Here's how the part is built. I have some questions about the finished solid (model axes, mm). Face numbers are marked on the shaded views. A direction names the side the tool comes from. Round coordinates to 2 decimals unless told otherwise and drop trailing zeros. Write each loop counter-clockwise with the first axis right and the second up, starting at its lowest first coordinate (ties: lowest second). Pieces come first, ordered by that corner, then holes. Notation, with made-up numbers: (6.5, 80.5) -> (60.5, 80.5) arc R16 cw to (60.5, 105.5) -> close; hole circle Ø5 at (76, 57). An arc over 180 degrees is marked (long way). Put each result on its own line as item: value. Start each with the question number.
1) I want a section at B-B, the plane z = -15.5. List the corners of the cut face in (x, y) for me.
2) I want a section at A-A, the plane x = 15.5. List the corners of the cut face in (y, z) for me, then the cut area to 3 significant figures.
3) Which directions (+Z, -Z, +X, -X, +Y, -Y) give clear straight access to the entire face, cutting with the end or side of a thin tool? Please do the marked faces 1, 2 and 3.
4) I want a section at C-C, the plane y = 3.4. List the corners of the cut face in (x, z) for me.
5) If I drill on line 1 along Z through (x, y) = (7.5, 3.2); line 2 along Z through (x, y) = (7.5, 1.75); line 3 along X through (y, z) = (2.9, -55), over which ranges is the centre line in solid material (lowest first)? Write a range as [from, to].
6) Will these pins go through, and if not, where does the flat tip stop? P1, Ø6, axis at x = 22.5, z = -40, coming from the +Y side; P2, Ø3, axis at y = 1.5, z = -19, coming from the -X side; P3, Ø1.2, axis at x = 2.5, y = 3.5, coming from the +Z side.
7) I want a section at D-D, the plane z = -55. List the corners of the cut face in (x, y) for me.
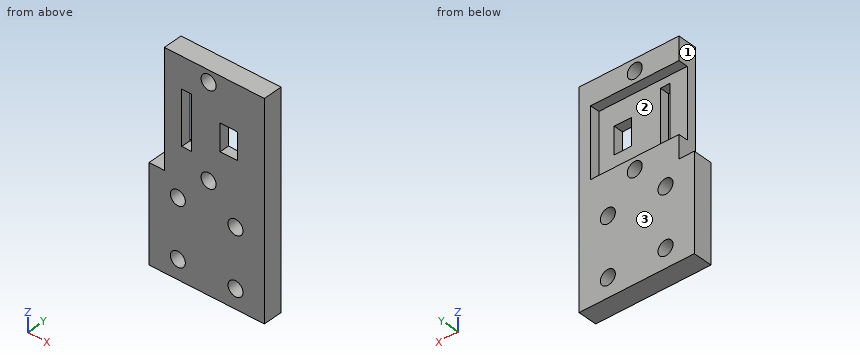
from build123d import *

# Parameters (mm, degrees)
ESQUISSE1_W             = 30
ESQUISSE1_H             = 60
BOSS_EXTRU_1_DEPTH      = 5
D_GAGEMENT_M3_51_D      = 3.9
ESQUISSE19_W            = 26
ESQUISSE19_H            = 5
ENL_V_MAT_EXTRU_5_DEPTH = 6
D_GAGEMENT_M3_53_D      = 3.9
D_GAGEMENT_M3_53_DEPTH  = 5
D_GAGEMENT_M3_53_TIP    = 1.171678207
ESQUISSE22_W            = 23
ESQUISSE22_H            = 18
ENL_V_MAT_EXTRU_6_DEPTH = 2.5
ESQUISSE23_W            = 2.5
ESQUISSE23_H            = 14
ESQUISSE23_W_2          = 4.5
ESQUISSE23_H_2          = 7
ENL_V_MAT_EXTRU_7_DEPTH = 3.5


with BuildPart() as part:
    # Esquisse1 → Boss.-Extru.1 (new body)
    with BuildSketch(Plane(origin=(0, 0, 0), x_dir=(1, 0, 0), z_dir=(0, 1, 0))):
        with Locations((15, 30)):
            Rectangle(ESQUISSE1_W, ESQUISSE1_H)
    extrude(amount=BOSS_EXTRU_1_DEPTH)

    # Dégagement M3.51 (through all)
    with Locations(Plane(origin=(0, 5, 0), x_dir=(1, 0, 0), z_dir=(0, 1, 0))):
        with Locations((7.5, 40), (22.5, 40), (22.5, 55), (7.5, 55)):
            Hole(D_GAGEMENT_M3_51_D / 2)

    # Esquisse19 → Enlèv. mat.-Extru.5 (cut, through all)
    with BuildSketch(Plane(origin=(0, 5, 0), x_dir=(1, 0, 0), z_dir=(0, 1, 0))):
        Polygon((4, 5), (4, 35), (0, 35), (0, 0), (4, 0), align=None)
        with Locations((17, 2.5)):
            Rectangle(ESQUISSE19_W, ESQUISSE19_H)
    extrude(amount=-ENL_V_MAT_EXTRU_5_DEPTH, mode=Mode.SUBTRACT)

    # Dégagement M3.53
    with Locations(Plane(origin=(0, 5, 0), x_dir=(1, 0, 0), z_dir=(0, 1, 0))):
        with Locations((15.5, 32), (15.5, 8)):
            Hole(D_GAGEMENT_M3_53_D / 2, depth=D_GAGEMENT_M3_53_DEPTH)
            with Locations((0, 0, -(D_GAGEMENT_M3_53_DEPTH + D_GAGEMENT_M3_53_TIP / 2))):  # 118° drill point
                Cone(0, D_GAGEMENT_M3_53_D / 2, D_GAGEMENT_M3_53_TIP, mode=Mode.SUBTRACT)

    # Esquisse22 → Enlèv. mat.-Extru.6 (cut)
    with BuildSketch(Plane(origin=(0, 5, 0), x_dir=(1, 0, 0), z_dir=(0, 1, 0))):
        with Locations((15.5, 20)):
            Rectangle(ESQUISSE22_W, ESQUISSE22_H)
    extrude(amount=-ENL_V_MAT_EXTRU_6_DEPTH, mode=Mode.SUBTRACT)

    # Esquisse23 → Enlèv. mat.-Extru.7 (cut, through all)
    with BuildSketch(Plane(origin=(0, 2.5, 0), x_dir=(1, 0, 0), z_dir=(0, 1, 0))):
        with Locations((9.75, 20)):
            Rectangle(ESQUISSE23_W, ESQUISSE23_H)
        with Locations((20.75, 20)):
            Rectangle(ESQUISSE23_W_2, ESQUISSE23_H_2)
    extrude(amount=-ENL_V_MAT_EXTRU_7_DEPTH, mode=Mode.SUBTRACT)


solid = part.part
Findings:
1. outline: (4, 0) -> (8.5, 0) -> (8.5, 2.5) -> (4, 2.5) -> close; (11, 0) -> (30, 0) -> (30, 5) -> (27, 5) -> (27, 2.5) -> (11, 2.5) -> close
2. outline: (0, -60) -> (5, -60) -> (5, -33.95) -> (0, -33.95) -> close; (0, -30.05) -> (5, -30.05) -> (5, -29) -> (2.5, -29) -> (2.5, -11) -> (5, -11) -> (5, -9.95) -> (0, -9.95) -> close; (0, -6.05) -> (5, -6.05) -> (5, -5) -> (0, -5) -> close
2. area: 191 mm2
3. face 1: +Z, -X, +Y, -Y
3. face 2: -X, +Y
3. face 3: +Z, -Z, +X, -X, +Y
4. outline: (0, -60) -> (30, -60) -> (30, -5) -> (4, -5) -> (4, -11) -> (27, -11) -> (27, -29) -> (4, -29) -> (4, -35) -> (0, -35) -> close; hole circle Ø3.9 at (7.5, -55); hole circle Ø3.9 at (7.5, -40); hole circle Ø3.9 at (15.5, -32); hole circle Ø3.9 at (15.5, -8); hole circle Ø3.9 at (22.5, -55); hole circle Ø3.9 at (22.5, -40)
5. line 1: z = [-60, -56.95], [-53.05, -41.95], [-38.05, -29], [-11, -5]
5. line 2: z = [-60, -56.95], [-53.05, -41.95], [-38.05, -5]
5. line 3: x = [0, 5.55], [9.45, 20.55], [24.45, 30]
6. P1: stops at y = 5
6. P2: stops at x = 4
6. P3: stops at z = -35
7. outline: (0, 0) -> (5.55, 0) -> (5.55, 5) -> (0, 5) -> close; (9.45, 0) -> (20.55, 0) -> (20.55, 5) -> (9.45, 5) -> close; (24.45, 0) -> (30, 0) -> (30, 5) -> (24.45, 5) -> close
